Here's how the part is built. I have some questions about the finished solid (model axes, mm). A direction names the side the tool comes from. Coordinates: 2 decimals unless noted, no trailing zeros. Loops run counter-clockwise (first coordinate to the right, second up) from the corner with the lowest first, then second, coordinate; pieces in that order, holes last.
Autodesk Inventor part; units mm, degrees
ref_plane "YZ Plane" through (0, 0, 0) normal (1, 0, 0) x (0, 1, 0)
ref_plane "XZ Plane" through (0, 0, 0) normal (0, 1, 0) x (-1, 0, 0)
ref_plane "XY Plane" through (0, 0, 0) normal (0, 0, 1) x (1, 0, 0)
sketch "草圖1" plane through (0, 0, 0) normal (0, 0, 1) x (1, 0, 0)
  line L0 (-29.4, 0) -> (29.4, 0)
  line L1 (0, -5.95) -> (0, 5.95)
  line L2 (-21, 4.25) -> (21, 4.25)
  line L3 (21, 4.25) -> (21, -4.25)
  line L4 (21, -4.25) -> (-21, -4.25)
  line L5 (-21, -4.25) -> (-21, 4.25)
  point P0 (0, 0)
  dimension "d0" = 8.5
  dimension "d1" = 42
extrude "擠出1" add sketch "草圖1" along normal blind 10
sketch "草圖2" plane through (-21, -4.25, 0) normal (0, -1, 0) x (1, 0, 0)
  line L0 (0, 0) -> (42, 0)
  line L1 (42, 0) -> (42, 10)
  line L2 (0, 10) -> (42, 10)
  line L3 (0, 0) -> (0, 10)
  circle A0 centre (10, 5) radius 4
  circle A1 centre (10, 5) radius 1.65
  line L4 (21, 0) -> (21, -1.5889)
  circle A2 centre (32, 5) radius 4
  circle A3 centre (32, 5) radius 1.65
  line L5 (10, 1.7091) -> (7.15, 3.3546)
  line L6 (7.15, 3.3546) -> (7.15, 6.6454)
  line L7 (7.15, 6.6454) -> (10, 8.2909)
  line L8 (10, 8.2909) -> (12.85, 6.6454)
  line L9 (12.85, 6.6454) -> (12.85, 3.3546)
  line L10 (12.85, 3.3546) -> (10, 1.7091)
  line L11 (32, 1.7091) -> (29.15, 3.3546)
  line L12 (29.15, 3.3546) -> (29.15, 6.6454)
  line L13 (29.15, 6.6454) -> (32, 8.2909)
  line L14 (32, 8.2909) -> (34.85, 6.6454)
  line L15 (34.85, 6.6454) -> (34.85, 3.3546)
  line L16 (34.85, 3.3546) -> (32, 1.7091)
  point P0 (29.15, 5)
  dimension "d5" = 3.3
  dimension "d6" = 10
  dimension "d24" = 5.7
  dimension "d25" = 5.7
  dimension "d32" = 5
extrude "擠出2" cut sketch "草圖2" against normal blind 10 contours A1 | A3
sketch "草圖3" plane through (0, 0, 10) normal (0, 0, 1) x (1, 0, 0)
  line L0 (-21, -4.25) -> (21, -4.25)
  line L1 (21, -4.25) -> (21, 4.25)
  line L2 (21, 4.25) -> (-21, 4.25)
  line L3 (-21, 4.25) -> (-21, -4.25)
  line L4 (-17.8, -4.25) -> (-21, -1.05)
  line L5 (0, 4.25) -> (0, 6.2817)
  line L6 (17.8, -4.25) -> (21, -1.05)
  line L7 (17.8, -4.25) -> (22.3255, -4.25) construction
  circle A0 centre (-15.5, 0.75) radius 1.65
  circle A1 centre (-15.5, 0.75) radius 3
  circle A2 centre (15.5, 0.75) radius 1.65
  circle A3 centre (15.5, 0.75) radius 3
  line L8 (-18.5, 0.75) -> (-12.5, 0.75)
  line L9 (-12.5, 0.75) -> (-12.5, 4.25)
  line L10 (-12.5, 4.25) -> (-18.5, 4.25)
  line L11 (-18.5, 4.25) -> (-18.5, 0.75)
  line L12 (12.5, 0.75) -> (18.5, 0.75)
  line L13 (18.5, 0.75) -> (18.5, 4.25)
  line L14 (18.5, 4.25) -> (12.5, 4.25)
  line L15 (12.5, 4.25) -> (12.5, 0.75)
  point P0 (0, 0)
  point P1 (13.85, 0.75)
  point P2 (17.15, 0.75)
  point P3 (12.5, 4.25)
  point P4 (-12.5, 0.75)
  point P5 (-17.15, 0.75)
  point P6 (-13.85, 0.75)
  dimension "d16" = 6
  dimension "d11" = 3.2
  dimension "d12" = 45
  dimension "d13" = 45
  dimension "d14" = 3.2
  dimension "d15" = 3.3
  dimension "d17" = 5.5
  dimension "d28" = 3.5
extrude "擠出4" cut sketch "草圖3" against normal up to surface (10 mm away) contours L3 L4 L0 | L6 L1 L0 | L8 A0 | A0 L8 | L12 A2 | A2 L12
extrude "擠出6" cut sketch "草圖3" against normal blind 2.3 contours L8 A0 A1 | A1 L8 A0 | A0 L8 | L12 A2 A3 | A3 L12 A2 | L12 A2 picked at (-15.1043, 1.2463) picked at (16.003, 1.1372)
extrude "擠出7" cut sketch "草圖2" against normal blind 3 contours A1 | A3 | L5 L6 L7 L8 L9 L10 | L11 L12 L13 L14 L15 L16
properties part number "y_motor_lock_bottom2_3D 列印"
1. I want a section at B-B (y = 0.75). Please give me the cut outline in (x, z), then the cut area to 3 significant figures.
2. On a 3-axis mill with a long thin cutter (end or side, diameter ignored), from which of +Z, -Z, +X, -X, +Y, -Y can I reach the whole of each face in a straight line? I mean faces 1 (the flat face through (-9.56, -2.77, 2.54)), 2 (the flat face through (17, -1, 7.7)), 3 (the cylindrical face through (-13.976, 0.118, 3.904)). Say none if no direction works.
3. We'd pull the mould along Z, two halves only. Please class faces 4 (the flat face through (0, 0, 0)), 5 (the flat face through (0, 0, 10)), 6 (the flat face through (-21, 2, 5)), 7 (the flat face through (-12.405, -2.771, 2.52)): +Z half, -Z half, draft (parallel to the pull), parting line (faces both ways), or undercut.
4. I want a section at C-C (x = 15.5). Please give me the cut outline in (y, z), then the cut area to 3 significant figures.
5. I want a section at A-A (z = 5). Please give me the cut outline in (x, y).
6. For pin 1 (2.5 mm diameter, centred on y = -2.5, z = 5.5, fed in from -X); pin 2 (0.9 mm diameter, centred on y = -3, z = 5, fed in from +X); pin 3 (3 mm diameter, centred on x = -11, z = 5, fed in from +Y); pin 4 (0.9 mm diameter, centred on y = -3.5, z = 5.5, fed in from -X), each with a flat end and sliding along its axis, tell me the tip position at first contact or that it passes through.
7. I want a section at D-D (x = -12). Please give me the cut outline in (y, z), then the cut area to 3 significant figures.
8. I need wall thicknesses on line 1 along X through (y, z) = (0.75, 9.3); line 2 along Z through (x, y) = (11, 0.2); line 3 along Y through (x, z) = (-15.5, 3.75). Which ranges of each line are inside material? Lowest first, please.
Response values:
1. outline: (-21, 0) - (-17.15, 0) - (-17.15, 7.7) - (-18.5, 7.7) - (-18.5, 10) - (-21, 10) - close; (-13.85, 0) - (13.85, 0) - (13.85, 7.7) - (12.5, 7.7) - (12.5, 10) - (-12.5, 10) - (-12.5, 7.7) - (-13.85, 7.7) - close; (17.15, 0) - (21, 0) - (21, 10) - (18.5, 10) - (18.5, 7.7) - (17.15, 7.7) - close; hole circle Ø3.3 at (-11, 5); hole circle Ø3.3 at (11, 5)
1. area: 324 mm2
2. face 1: -Y
2. face 2: +Z
2. face 3: +Z, -Z
3. face 4: -Z half
3. face 5: +Z half
3. face 6: draft
3. face 7: undercut
4. outline: (-4.25, 0) - (-0.9, 0) - (-0.9, 7.7) - (-2.25, 7.7) - (-2.25, 10) - (-4.25, 10) - close; (2.4, 0) - (4.25, 0) - (4.25, 10) - (3.75, 10) - (3.75, 7.7) - (2.4, 7.7) - close
4. area: 45.8 mm2
5. outline: (-21, -1.05) - (-17.8, -4.25) - (-13.85, -4.25) - (-13.85, -1.25) - (-12.65, -1.25) - (-12.65, 4.25) - (-21, 4.25) - close; (-9.35, -1.25) - (-8.15, -1.25) - (-8.15, -4.25) - (8.15, -4.25) - (8.15, -1.25) - (9.35, -1.25) - (9.35, 4.25) - (-9.35, 4.25) - close; (12.65, -1.25) - (13.85, -1.25) - (13.85, -4.25) - (17.8, -4.25) - (21, -1.05) - (21, 4.25) - (12.65, 4.25) - close; hole circle Ø3.3 at (-15.5, 0.75); hole circle Ø3.3 at (15.5, 0.75)
6. pin 1: stops at x = -20.8
6. pin 2: stops at x = 19.5
6. pin 3: passes through
6. pin 4: stops at x = -19
7. outline: (-4.25, 0) - (4.25, 0) - (4.25, 3.69) - (-1.25, 3.69) - (-1.25, 2.29) - (-4.25, 2.29) - close; (-4.25, 7.71) - (-1.25, 7.71) - (-1.25, 6.31) - (4.25, 6.31) - (4.25, 10) - (-4.25, 10) - close
7. area: 54.3 mm2
8. line 1: x = -21 to -18.5, -12.5 to 12.5, 18.5 to 21
8. line 2: z = 0 to 3.35, 6.65 to 10
8. line 3: y = -4.25 to -0.9, 2.4 to 4.25
